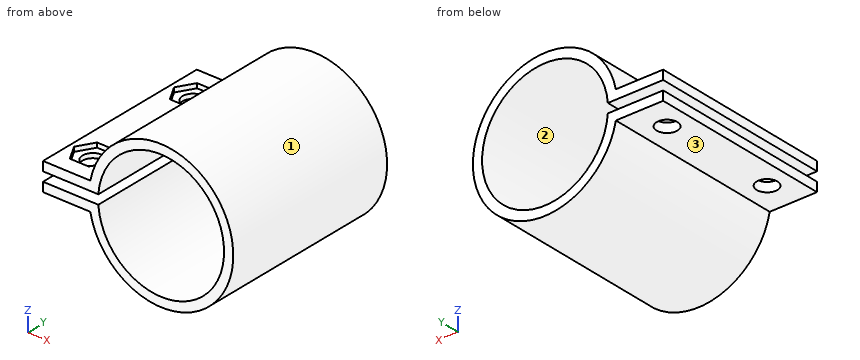
from build123d import *

# Parameters (mm, degrees)
F1_DEPTH = 40
F3_DEPTH = 1
F4_R     = 2.25
F5_DEPTH = 18.701


with BuildPart() as f1:
    # F0 (on Front) → F1 (new body)
    with BuildSketch(Plane.XZ):
        with BuildLine():
            ThreePointArc((-13.663455, 1), (13.7, 0), (-13.663455, -1))
            Line((-13.663455, -1), (-25.7, -1))
            Line((-25.7, -1), (-25.7, -3))
            Line((-25.7, -3), (-15.410711, -3))
            ThreePointArc((-15.410711, -3), (15.7, 0), (-15.410711, 3))
            Line((-15.410711, 3), (-25.7, 3))
            Line((-25.7, 3), (-25.7, 1))
            Line((-25.7, 1), (-13.663455, 1))
        make_face()
    extrude(amount=F1_DEPTH)

    # F2 (on face) → F3 (cut)
    with BuildSketch(Plane.XY.offset(3)):
        Polygon((-16.600813, -33), (-18.650407, -29.45), (-22.749593, -29.45), (-24.799187, -33), (-22.749593, -36.55), (-18.650407, -36.55), align=None)
        Polygon((-24.799187, -7), (-22.749593, -10.55), (-18.650407, -10.55), (-16.600813, -7), (-18.650407, -3.45), (-22.749593, -3.45), align=None)
    extrude(amount=-F3_DEPTH, mode=Mode.SUBTRACT)

    # F4 (on face) → F5 (cut, through all)
    with BuildSketch(Plane.XY.offset(3)):
        with Locations((-20.7, -33)):
            Circle(F4_R)
        with Locations((-20.7, -7)):
            Circle(F4_R)
    extrude(amount=-F5_DEPTH, mode=Mode.SUBTRACT)


solid = f1.part
For this review, take the finished solid that the model builds, in its own axes (mm). Face numbers are marked on the shaded views. Give positions to 0.01 mm unless a question says otherwise; leave off trailing zeros. Loops run counter-clockwise (first coordinate to the right, second up) from the corner with the lowest first, then second, coordinate; pieces in that order, holes last. Notation, with made-up numbers: (35.25, -14) - (50.25, -14) arc R26 ccw to (50.25, 3) - close; hole circle Ø10 at (-37, 27). An arc over 180 degrees is marked (long way). Write each question's results on one line, items separated by ' | '.
(1) Take a section at D-D (z = -9.5). Give the boundary of the cut face in (x, y).
Conclusion:
outline: (-12.5, -40) - (-9.87, -40) - (-9.87, 0) - (-12.5, 0) - close; (9.87, -40) - (12.5, -40) - (12.5, 0) - (9.87, 0) - close
(2) Take a section at B-B (x = 0). Give the boundary of the cut face in (y, z).
Conclusion:
outline: (-40, -15.7) - (0, -15.7) - (0, -13.7) - (-40, -13.7) - close; (-40, 13.7) - (0, 13.7) - (0, 15.7) - (-40, 15.7) - close
(3) Draft analysis for pull direction X (two halves, no side actions). For the marked faces 1, 2 and 3, state which applies: +X half, -X half, draft (parallel to the pull), parting line (faces both ways), or undercut.
Conclusion:
face 1: parting line | face 2: undercut | face 3: draft
(4) Take a section at C-C (y = -34.5). Give the boundary of the cut face in (x, z), then the cut area to 3 significant figures.
Conclusion:
outline: (-25.7, -3) - (-22.38, -3) - (-22.38, -1) - (-25.7, -1) - close; (-25.7, 1) - (-22.38, 1) - (-22.38, 2) - (-23.93, 2) - (-23.93, 3) - (-25.7, 3) - close; (-19.02, -3) - (-15.41, -3) arc R15.7 ccw (long way) to (-15.41, 3) - (-17.47, 3) - (-17.47, 2) - (-19.02, 2) - (-19.02, 1) - (-13.66, 1) arc R13.7 cw (long way) to (-13.66, -1) - (-19.02, -1) - close | area: 205 mm^2
(5) Take a section at A-A (x = -20.7). State how many separate pieces and enclosed holes the cut face has, then the cut area to 3 significant figures.
Conclusion:
separate pieces: 6 | enclosed holes: 0 | area: 119 mm^2
(6) For pin 1 Ø12 at (x, y) = (-18.5, -8) entering from +Z; pin 2 Ø8 at (x, y) = (-21.5, -7.5) entering from +Z; pin 3 Ø4 at (y, z) = (-6.5, -10.5) entering from +X; pin 4 Ø2 at (x, y) = (-21, -8) entering from +Z, all flat-tipped, find the tip position at first contact; note any pin that passes through.
Conclusion:
pin 1: z = 9.5 | pin 2: z = 3 | pin 3: x = 13.2 | pin 4: through
(7) For line 1 along Y through (x, z) = (-20.7, -2.1); line 2 along Z through (x, y) = (0, -17); line 3 along Y through (x, z) = (-20, -2), list the stretches that pass through material, from the lowest coordinate up.
Conclusion:
line 1: -40 to -35.25, -30.75 to -9.25, -4.75 to 0 | line 2: -15.7 to -13.7, 13.7 to 15.7 | line 3: -40 to -35.14, -30.86 to -9.14, -4.86 to 0
